```python
from build123d import *

# Parameters (mm, degrees)
ESQUISSE1_R                      = 90
BOSS_EXTRU_1_DEPTH               = 50
ESQUISSE2_R                      = 70
ENL_V_MAT_EXTRU_1_DEPTH          = 10
ESQUISSE3_R                      = 150
BOSS_EXTRU_2_DEPTH               = 20
ESQUISSE4_R                      = 15
ENL_V_MAT_EXTRU_2_DEPTH          = 10
R_P_TITION_START                 = 60
R_P_TITION_CIRCULAIRE1_OUTLINE_R = 15
R_P_TITION_CIRCULAIRE1_DEPTH     = 10


# Read off the part's stored shape, not the designer's step: Répétition circulaire1
with BuildPart() as part:
    # Esquisse1 → Boss.-Extru.1 (new body)
    with BuildSketch(Plane(origin=(0, 0, 0), x_dir=(1, 0, 0), z_dir=(0, 1, 0))):
        with Locations(Location((0, 0, 0), (0, 0, 270))):
            Circle(ESQUISSE1_R)
    extrude(amount=BOSS_EXTRU_1_DEPTH)

    # Esquisse2 → Enlèv. mat.-Extru.1 (cut)
    with BuildSketch(Plane(origin=(0, 0, 0), x_dir=(-1, 0, 0), z_dir=(0, -1, 0))):
        with Locations(Location((0, 0, 0), (0, 0, 90))):
            Circle(ESQUISSE2_R)
    extrude(amount=-ENL_V_MAT_EXTRU_1_DEPTH, mode=Mode.SUBTRACT)

    # Esquisse3 → Boss.-Extru.2 (add)
    with BuildSketch(Plane(origin=(0, 50, 0), x_dir=(1, 0, 0), z_dir=(0, 1, 0))):
        with Locations(Location((0, 0, 0), (0, 0, 270))):
            Circle(ESQUISSE3_R)
    extrude(amount=BOSS_EXTRU_2_DEPTH)

    # Esquisse4 → Enlèv. mat.-Extru.2 (cut)
    with BuildSketch(Plane(origin=(0, 70, 0), x_dir=(1, 0, 0), z_dir=(0, 1, 0))):
        with Locations(Location((-125, 0, 0), (0, 0, 270))):
            Circle(ESQUISSE4_R)
    extrude(amount=-ENL_V_MAT_EXTRU_2_DEPTH, mode=Mode.SUBTRACT)

    # Répétition circulaire1 outline → Répétition circulaire1 (cut)
    with BuildSketch(Plane(origin=(0, 0, 0), x_dir=(1, 0, 0), z_dir=(0, 1, 0)).offset(R_P_TITION_START)):
        with Locations((-117.385431917, -43.184361531)):
            Circle(R_P_TITION_CIRCULAIRE1_OUTLINE_R)
        with Locations((-117.385431917, 43.184361531)):
            Circle(R_P_TITION_CIRCULAIRE1_OUTLINE_R)
        with Locations((-95.460156959, 81.160051728)):
            Circle(R_P_TITION_CIRCULAIRE1_OUTLINE_R)
        with Locations((-61.868686869, 109.346641892)):
            Circle(R_P_TITION_CIRCULAIRE1_OUTLINE_R)
        with Locations((-20.662648695, 124.344413259)):
            Circle(R_P_TITION_CIRCULAIRE1_OUTLINE_R)
        with Locations((23.187901221, 124.344413259)):
            Circle(R_P_TITION_CIRCULAIRE1_OUTLINE_R)
        with Locations((64.393939394, 109.346641892)):
            Circle(R_P_TITION_CIRCULAIRE1_OUTLINE_R)
        with Locations((97.985409485, 81.160051728)):
            Circle(R_P_TITION_CIRCULAIRE1_OUTLINE_R)
        with Locations((119.910684443, 43.184361531)):
            Circle(R_P_TITION_CIRCULAIRE1_OUTLINE_R)
        with Locations((127.525252525, 0)):
            Circle(R_P_TITION_CIRCULAIRE1_OUTLINE_R)
        with Locations((119.910684443, -43.184361531)):
            Circle(R_P_TITION_CIRCULAIRE1_OUTLINE_R)
        with Locations((97.985409485, -81.160051728)):
            Circle(R_P_TITION_CIRCULAIRE1_OUTLINE_R)
        with Locations((64.393939394, -109.346641892)):
            Circle(R_P_TITION_CIRCULAIRE1_OUTLINE_R)
        with Locations((23.187901221, -124.344413259)):
            Circle(R_P_TITION_CIRCULAIRE1_OUTLINE_R)
        with Locations((-20.662648695, -124.344413259)):
            Circle(R_P_TITION_CIRCULAIRE1_OUTLINE_R)
        with Locations((-61.868686869, -109.346641892)):
            Circle(R_P_TITION_CIRCULAIRE1_OUTLINE_R)
        with Locations((-95.460156959, -81.160051728)):
            Circle(R_P_TITION_CIRCULAIRE1_OUTLINE_R)
    extrude(amount=R_P_TITION_CIRCULAIRE1_DEPTH, mode=Mode.SUBTRACT)


solid = part.part
```
The listing builds one solid part. Answer for the finished solid, in the listing's coordinates (mm). A direction names the side the tool comes from. Coordinates: 2 decimals unless noted, no trailing zeros. Write each loop counter-clockwise with the first axis right and the second up, starting at its lowest first coordinate (ties: lowest second). Pieces come first, ordered by that corner, then holes. Notation, with made-up numbers: (33, 33) -> (49, 33) arc R30 ccw to (49, 58) -> close; hole circle Ø7 at (-22, 82.5). An arc over 180 degrees is marked (long way). Write each question's results on one line, items separated by ' | '. Start each with the question number.
1) A cutting plane is placed at B-B (z = 0). Determine the outline of the cut face in (x, y).
2) A cutting plane is placed at D-D (x = -125). Determine the outline of the cut face in (y, z), then the cut area to 3 significant figures.
3) For a pull along Z with two mould halves and no side action, classify faces 1 (the flat face through (120, 60, 43)), 2 (the flat face through (-65, 50, 65)) as +Z half, -Z half, draft (parallel to the pull), parting line (faces both ways), or undercut.
4) A cutting plane is placed at A-A (x = 0). Determine the outline of the cut face in (y, z).
5) Flat-ended cylindrical pins translate along their axes: pin 1 Ø3 at (y, z) = (23, 83.5) entering from -X; pin 2 Ø9 at (x, z) = (-56.5, -106.5) entering from +Y; pin 3 Ø2 at (x, y) = (-70, 58) entering from -Z. Find the tip coordinate at first contact, or state that the pin passes through.
6) A cutting plane is placed at C-C (y = 37.5). Determine the outline of the cut face in (x, z).
7) Straight lines are drawn through the part: probe 1 along Z at (x, y) = (11, 65); probe 2 along Z at (x, y) = (58, 64); probe 3 along X at (y, z) = (62.5, -97.5). For each, find the intervals that lie inside material, in ascending order.
8) A tool of negligible diameter and unlimited length cuts with its end or side. For faces 3 (the flat face through (-118, 60, -43)), 4 (the flat face through (1, 10, 1)), 5 (the flat face through (2, 70, -2)), from which of +Z, -Z, +X, -X, +Y, -Y can it reach the whole face along a straight path? Write none if from no direction.
Values follow:
1) outline: (-150, 50) -> (-90, 50) -> (-90, 0) -> (-70, 0) -> (-70, 10) -> (70, 10) -> (70, 0) -> (90, 0) -> (90, 50) -> (150, 50) -> (150, 70) -> (142.53, 70) -> (142.53, 60) -> (112.53, 60) -> (112.53, 70) -> (-110, 70) -> (-110, 60) -> (-140, 60) -> (-140, 70) -> (-150, 70) -> close
2) outline: (50, -82.92) -> (70, -82.92) -> (70, -56.11) -> (60, -56.11) -> (60, -30.26) -> (70, -30.26) -> (70, -15) -> (60, -15) -> (60, 15) -> (70, 15) -> (70, 30.26) -> (60, 30.26) -> (60, 56.11) -> (70, 56.11) -> (70, 82.92) -> (50, 82.92) -> close | area: 2,500 mm²
3) face 1: undercut | face 2: draft
4) outline: (0, -90) -> (50, -90) -> (50, -150) -> (70, -150) -> (70, 150) -> (50, 150) -> (50, 90) -> (0, 90) -> (0, 70) -> (10, 70) -> (10, -70) -> (0, -70) -> close
5) pin 1: x = -37.09 | pin 2: y = 60 | pin 3: z = -133.19
6) outline: circle Ø180 at (0, 0)
7) probe 1: -149.6 to -133.09, -115.6 to 115.6, 133.09 to 149.6 | probe 2: -138.33 to -122.92, -95.78 to 95.78, 122.92 to 138.33 | probe 3: -113.99 to -71.07, -52.67 to 55.19, 73.59 to 113.99
8) face 3: +Y | face 4: -Y | face 5: +Z, -Z, +X, -X, +Y
